Design review of the part built by this model. Coordinates are the model's own, in mm. Give positions to 0.01 mm unless a question says otherwise; leave off trailing zeros. Loops run counter-clockwise (first coordinate to the right, second up) from the corner with the lowest first, then second, coordinate; pieces in that order, holes last. Notation, with made-up numbers: (73.25, -24) -> (90.25, -24) arc R29 cw to (90.25, 11) -> close; hole circle Ø4 at (88.5, -25.75). An arc over 180 degrees is marked (long way). Answer in a Markdown table with one row per item. Add a question column.
(1) For line 1 (Z direction, x = 121, y = 2.6); line 2 (X direction, y = 2.1, z = -40); line 3 (X direction, y = 1.35, z = -34), list the stretches that pass through material, from the lowest coordinate up.
(2) Consider section C-C on y = 1. Count the separate pieces of the cut face and the enclosed holes in it, then the cut area to 3 significant figures.
(3) Consider section A-A on x = 135.5. Write out the cut boundary in (y, z).
(4) For pin 1 (21 mm diameter, centred on x = 25.98, z = -34.8, fed in from +Y), flat-tipped, find the tip position at first contact; note if it passes through.
(5) Consider section B-B on z = -30. Write out the cut boundary in (x, y).
(6) Consider section D-D on z = -38. Write out the cut boundary in (x, y).
from build123d import *

# Parameters (mm, degrees)
SKETCH1_W                = 150
SKETCH1_H                = 70
BOSS_EXTRUDE1_DEPTH      = 3
SKETCH2_R                = 13
SKETCH2_R_2              = 0.8
CUT_EXTRUDE1_DEPTH       = 166.556636835
SKETCH3_R                = 13
CUT_EXTRUDE2_DEPTH       = 1
M3_CLEARANCE_HOLE1_D     = 3.4
M3_CLEARANCE_HOLE1_DEPTH = 7
M3_CLEARANCE_HOLE1_TIP   = 1.021463052


with BuildPart() as part:
    # Sketch1 → Boss-Extrude1 (new body)
    with BuildSketch(Plane(origin=(0, 0, 0), x_dir=(1, 0, 0), z_dir=(0, 1, 0))):
        with Locations((75, 35)):
            Rectangle(SKETCH1_W, SKETCH1_H)
    extrude(amount=BOSS_EXTRUDE1_DEPTH)

    # Sketch2 → Cut-Extrude1 (cut, through all)
    with BuildSketch(Plane(origin=(0, 3, 0), x_dir=(1, 0, 0), z_dir=(0, 1, 0))):
        with Locations(Location((125.978759571, 34.795735311, 0), (0, 0, 270))):
            Circle(SKETCH2_R)
        with Locations(Location((13.498759571, 43.695735311, 0), (0, 0, 270))):
            Circle(SKETCH2_R_2)
        with Locations(Location((13.498759571, 25.895735311, 0), (0, 0, 90))):
            Circle(SKETCH2_R_2)
        with BuildLine():
            Line((56.404199608, 44.795735311), (56.404199608, 24.795735311))
            ThreePointArc((56.404199608, 24.795735311), (54.404199608, 22.795735311), (52.404199608, 24.795735311))
            Line((52.404199608, 24.795735311), (52.404199608, 44.795735311))
            ThreePointArc((52.404199608, 44.795735311), (54.404199608, 46.795735311), (56.404199608, 44.795735311))
        make_face()
        with BuildLine():
            Line((18.498759571, 41.595735311), (11.828015738, 41.595735311))
            ThreePointArc((11.828015738, 41.595735311), (10.256762989, 34.795735311), (11.828015738, 27.995735311))
            Line((11.828015738, 27.995735311), (18.498759571, 27.995735311))
            ThreePointArc((18.498759571, 27.995735311), (36.08768632, 34.795735311), (18.498759571, 41.595735311))
        make_face()
    extrude(amount=-CUT_EXTRUDE1_DEPTH, mode=Mode.SUBTRACT)

    # Sketch3 → Cut-Extrude2 (cut)
    with BuildSketch(Plane(origin=(0, 3, 0), x_dir=(1, 0, 0), z_dir=(0, 1, 0))):
        with Locations((25.978759571, 34.795735311)):
            Circle(SKETCH3_R)
    extrude(amount=-CUT_EXTRUDE2_DEPTH, mode=Mode.SUBTRACT)

    # M3 Clearance Hole1
    with Locations(Plane(origin=(0, 3, 0), x_dir=(1, 0, 0), z_dir=(0, 1, 0))):
        with Locations((143.478759571, 34.795735311), (125.978759571, 52.295735311), (108.478759571, 34.795735311), (125.978759571, 17.295735311)):
            Hole(M3_CLEARANCE_HOLE1_D / 2, depth=M3_CLEARANCE_HOLE1_DEPTH)
            with Locations((0, 0, -(M3_CLEARANCE_HOLE1_DEPTH + M3_CLEARANCE_HOLE1_TIP / 2))):  # 118° drill point
                Cone(0, M3_CLEARANCE_HOLE1_D / 2, M3_CLEARANCE_HOLE1_TIP, mode=Mode.SUBTRACT)


solid = part.part
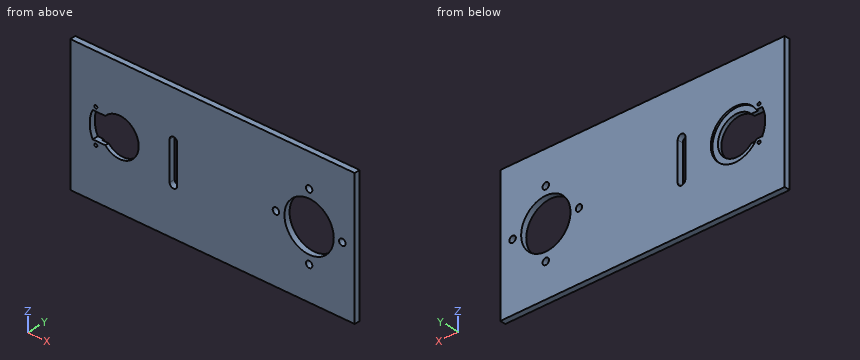
Values follow:
| question | item | result |
|---|---|---|
| 1 | line 1 | -70 to -46.8, -22.79 to 0 |
| 1 | line 2 | 0 to 11.16, 37.89 to 52.4, 56.4 to 114.07, 137.89 to 150 |
| 1 | line 3 | 0 to 10.28, 36.06 to 52.4, 56.4 to 106.98, 109.98 to 113, 138.95 to 141.98, 144.98 to 150 |
| 2 | separate pieces | 1 |
| 2 | enclosed holes | 9 |
| 2 | area | 9,430 mm2 |
| 3 | outline | (0, -70) -> (3, -70) -> (3, -43.65) -> (0, -43.65) -> close; (0, -25.94) -> (3, -25.94) -> (3, 0) -> (0, 0) -> close |
| 4 | pin 1 | y = 2 |
| 5 | outline | (0, 0) -> (11.02, 0) -> (11.02, 3) -> (0, 3) -> close; (34.88, 0) -> (52.4, 0) -> (52.4, 3) -> (38.06, 3) -> (38.06, 2) -> (34.88, 2) -> close; (56.4, 0) -> (113.9, 0) -> (113.9, 3) -> (56.4, 3) -> close; (138.06, 0) -> (150, 0) -> (150, 3) -> (138.06, 3) -> close |
| 6 | outline | (0, 0) -> (10.59, 0) -> (10.59, 3) -> (0, 3) -> close; (35.57, 0) -> (52.4, 0) -> (52.4, 3) -> (38.58, 3) -> (38.58, 2) -> (35.57, 2) -> close; (56.4, 0) -> (113.38, 0) -> (113.38, 3) -> (56.4, 3) -> close; (138.58, 0) -> (150, 0) -> (150, 3) -> (138.58, 3) -> close |
